CAD build for the part. Positions are in the model's coordinates, mm. Round coordinates to 2 decimals unless told otherwise and drop trailing zeros. Loops run counter-clockwise (first coordinate to the right, second up) from the corner with the lowest first, then second, coordinate; pieces in that order, holes last. Notation, with made-up numbers: (50, 7.25) - (59, 7.25) arc R30 ccw to (59, 42.25) - close; hole circle Ø6 at (68, 20.25). An arc over 180 degrees is marked (long way). One line per question, with ' | ' between items.
```python
from build123d import *

# Parameters (mm, degrees)
SKETCH_1_W            = 74
SKETCH_1_H            = 50
EXTRUDE_1_DEPTH       = 4
CUT_EXTRUDE_1_DEPTH   = 63.787339488
MIRROR_2_COPY_1_DEPTH = 63.787339488
SKETCH_3_R            = 13
CUT_EXTRUDE_2_DEPTH   = 63.787339488
FILLET_1_R            = 10
SKETCH_4_W            = 84
SKETCH_4_H            = 62
EXTRUDE_2_DEPTH       = 4
SKETCH_6_W            = 18
SKETCH_6_H            = 44
EXTRUDE_3_DEPTH       = 4
SKETCH_7_W            = 64
SKETCH_7_H            = 22
CUT_EXTRUDE_4_DEPTH   = 125.049385327
SKETCH_8_R            = 1.5
CUT_EXTRUDE_5_DEPTH   = 125.049385327
SKETCH_9_R            = 1.5
CUT_EXTRUDE_6_DEPTH   = 125.049385327
SKETCH_10_R           = 1.5
CUT_EXTRUDE_7_DEPTH   = 125.049385327
FILLET_2_R            = 3
SKETCH_11_W           = 20
SKETCH_11_H           = 18
CUT_EXTRUDE_8_DEPTH   = 125.049385327
FILLET_3_R            = 3
SKETCH_12_W           = 122.856865441
SKETCH_12_H           = 61.545901124
CUT_EXTRUDE_9_DEPTH   = 125.049385327
FILLET_4_R            = 3
FILLET_5_R            = 3
SKETCH_13_R           = 1.5
CUT_EXTRUDE_10_DEPTH  = 92.149602303
SKETCH_14_W           = 150.805924756
SKETCH_14_H           = 61.126695491
CUT_EXTRUDE_11_DEPTH  = 92.149602303
FILLET_6_R            = 1


with BuildPart() as part:
    # 草图1 → 凸台-拉伸1 (new body)
    with BuildSketch(Plane.XY):
        Polygon((37, 25), (42, 46.5), (-42, 46.5), (-37, 25), align=None)
        Rectangle(SKETCH_1_W, SKETCH_1_H)
    extrude(amount=EXTRUDE_1_DEPTH)

    # 草图2 → 切除-拉伸1 (cut, through all)
    with BuildSketch(Plane.XY.offset(4)):
        with BuildLine():
            ThreePointArc((29.5, 15), (29.939339828, 13.939339828), (31, 13.5))
            Line((31, 13.5), (31, 15))
            Line((31, 15), (29.5, 15))
        make_face()
        with BuildLine():
            Line((31, 15), (31, 13.5))
            ThreePointArc((31, 13.5), (32.060660172, 13.939339828), (32.5, 15))
            ThreePointArc((32.5, 15), (31, 16.5), (29.5, 15))
            Line((29.5, 15), (31, 15))
        make_face()
    cut_extrude_1 = extrude(amount=-CUT_EXTRUDE_1_DEPTH, mode=Mode.SUBTRACT)

    # 镜向1: 切除-拉伸1 across plane
    add(cut_extrude_1.mirror(Plane.ZX), mode=Mode.SUBTRACT)

    # 镜向2: 切除-拉伸1 across plane
    add(cut_extrude_1.mirror(Plane(origin=(0, 0, 0), x_dir=(0, 0, 1), z_dir=(1, 0, 0))), mode=Mode.SUBTRACT)

    # 镜向2 copy 1 sketch → 镜向2 copy 1 (cut, through all)
    with BuildSketch(Plane(origin=(0, 0, 4), x_dir=(-1, 0, 0), z_dir=(0, 0, 1))):
        with BuildLine():
            ThreePointArc((29.5, 15), (29.939339828, 13.939339828), (31, 13.5))
            Line((31, 13.5), (31, 15))
            Line((31, 15), (29.5, 15))
        make_face()
        with BuildLine():
            Line((31, 15), (31, 13.5))
            ThreePointArc((31, 13.5), (32.060660172, 13.939339828), (32.5, 15))
            ThreePointArc((32.5, 15), (31, 16.5), (29.5, 15))
            Line((29.5, 15), (31, 15))
        make_face()
    extrude(amount=-MIRROR_2_COPY_1_DEPTH, mode=Mode.SUBTRACT)

    # 草图3 → 切除-拉伸2 (cut, through all)
    with BuildSketch(Plane.XY.offset(4)):
        Circle(SKETCH_3_R)
    extrude(amount=-CUT_EXTRUDE_2_DEPTH, mode=Mode.SUBTRACT)

    # 圆角1
    fillet_1_edges = [part.edges().sort_by_distance(p)[0] for p in [
        (37, 25, 2),
        (-37, 25, 2),
    ]]
    fillet(fillet_1_edges, radius=FILLET_1_R)

    # 草图4 → 凸台-拉伸2 (add)
    with BuildSketch(Plane.XY.offset(4)):
        with Locations((0, 77.5)):
            Rectangle(SKETCH_4_W, SKETCH_4_H)
    extrude(amount=-EXTRUDE_2_DEPTH)

    # 草图6 → 凸台-拉伸3 (add)
    with BuildSketch(Plane.XY.offset(4)):
        with Locations((-51, 68.5)):
            Rectangle(SKETCH_6_W, SKETCH_6_H)
    extrude_3 = extrude(amount=-EXTRUDE_3_DEPTH)

    # 镜向4: 凸台-拉伸3 across plane
    add(extrude_3.mirror(Plane(origin=(0, 0, 0), x_dir=(0, 0, 1), z_dir=(1, 0, 0))))

    # 草图7 → 切除-拉伸4 (cut, through all)
    with BuildSketch(Plane.XY.offset(4)):
        with Locations((0, 69.5)):
            Rectangle(SKETCH_7_W, SKETCH_7_H)
    extrude(amount=-CUT_EXTRUDE_4_DEPTH, mode=Mode.SUBTRACT)

    # 草图8 → 切除-拉伸5 (cut, through all)
    with BuildSketch(Plane.XY.offset(4)):
        with Locations((0, 101)):
            Circle(SKETCH_8_R)
        with Locations((-24, 101)):
            Circle(SKETCH_8_R)
    cut_extrude_5 = extrude(amount=-CUT_EXTRUDE_5_DEPTH, mode=Mode.SUBTRACT)

    # 镜向5: 切除-拉伸5 across plane
    add(cut_extrude_5.mirror(Plane(origin=(0, 0, 0), x_dir=(0, 0, 1), z_dir=(1, 0, 0))), mode=Mode.SUBTRACT)

    # 草图9 → 切除-拉伸6 (cut, through all)
    with BuildSketch(Plane(origin=(0, 0, 0), x_dir=(-1, 0, 0), z_dir=(0, 0, -1))):
        with Locations((-52.5, 83.5)):
            Circle(SKETCH_9_R)
        with Locations((-52.5, 61)):
            Circle(SKETCH_9_R)
    cut_extrude_6 = extrude(amount=-CUT_EXTRUDE_6_DEPTH, mode=Mode.SUBTRACT)

    # 镜向6: 切除-拉伸6 across plane
    add(cut_extrude_6.mirror(Plane(origin=(0, 0, 0), x_dir=(0, 0, 1), z_dir=(1, 0, 0))), mode=Mode.SUBTRACT)

    # 草图10 → 切除-拉伸7 (cut, through all)
    with BuildSketch(Plane(origin=(0, 0, 0), x_dir=(-1, 0, 0), z_dir=(0, 0, -1))):
        with Locations((-30, 36)):
            Circle(SKETCH_10_R)
    cut_extrude_7 = extrude(amount=-CUT_EXTRUDE_7_DEPTH, mode=Mode.SUBTRACT)

    # 镜向7: 切除-拉伸7 across plane
    add(cut_extrude_7.mirror(Plane(origin=(0, 0, 0), x_dir=(0, 0, 1), z_dir=(1, 0, 0))), mode=Mode.SUBTRACT)

    # 圆角2
    fillet_2_edges = [part.edges().sort_by_distance(p)[0] for p in [
        (32, 80.5, 2),
        (32, 58.5, 2),
        (-32, 58.5, 2),
        (-32, 80.5, 2),
        (-42, 46.5, 2),
        (42, 46.5, 2),
        (-42, 90.5, 2),
        (42, 90.5, 2),
    ]]
    fillet(fillet_2_edges, radius=FILLET_2_R)

    # 草图11 → 切除-拉伸8 (cut, through all)
    with BuildSketch(Plane(origin=(0, 0, 0), x_dir=(-1, 0, 0), z_dir=(0, 0, -1))):
        with Locations((-50, 99.5)):
            Rectangle(SKETCH_11_W, SKETCH_11_H)
    cut_extrude_8 = extrude(amount=-CUT_EXTRUDE_8_DEPTH, mode=Mode.SUBTRACT)

    # 镜向8: 切除-拉伸8 across plane
    add(cut_extrude_8.mirror(Plane(origin=(0, 0, 0), x_dir=(0, 0, 1), z_dir=(1, 0, 0))), mode=Mode.SUBTRACT)

    # 圆角3
    fillet_3_edges = [part.edges().sort_by_distance(p)[0] for p in [
        (40, 90.5, 2),
        (-40, 90.5, 2),
    ]]
    fillet(fillet_3_edges, radius=FILLET_3_R)

    # 草图12 → 切除-拉伸9 (cut, through all)
    with BuildSketch(Plane(origin=(0, 0, 0), x_dir=(-1, 0, 0), z_dir=(0, 0, -1))):
        with Locations((1.42843272, 99.272950562)):
            Rectangle(SKETCH_12_W, SKETCH_12_H)
    extrude(amount=-CUT_EXTRUDE_9_DEPTH, mode=Mode.SUBTRACT)

    # 圆角4
    fillet_4_edges = [part.edges().sort_by_distance(p)[0] for p in [
        (-32, 68.5, 2),
        (32, 68.5, 2),
    ]]
    fillet(fillet_4_edges, radius=FILLET_4_R)

    # 圆角5
    fillet_5_edges = [part.edges().sort_by_distance(p)[0] for p in [
        (37, -25, 2),
        (-37, -25, 2),
    ]]
    fillet(fillet_5_edges, radius=FILLET_5_R)

    # 草图13 → 切除-拉伸10 (cut, through all)
    with BuildSketch(Plane.XY.offset(4)):
        with Locations((0, 36)):
            Circle(SKETCH_13_R)
    extrude(amount=-CUT_EXTRUDE_10_DEPTH, mode=Mode.SUBTRACT)

    # 草图14 → 切除-拉伸11 (cut, through all)
    with BuildSketch(Plane.XY.offset(4)):
        with Locations((-9.796052063, 74.063347746)):
            Rectangle(SKETCH_14_W, SKETCH_14_H)
    extrude(amount=-CUT_EXTRUDE_11_DEPTH, mode=Mode.SUBTRACT)

    # 圆角6
    fillet_6_edges = [part.edges().sort_by_distance(p)[0] for p in [
        (-41.302325581, 43.5, 2),
        (41.302325581, 43.5, 2),
    ]]
    fillet(fillet_6_edges, radius=FILLET_6_R)


solid = part.part
```
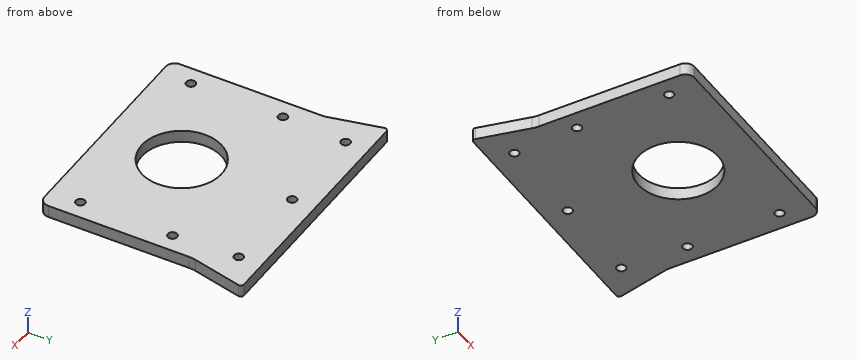
(1) Cut at B-B, the plane z = 1.05. State how many separate pieces and enclosed holes the cut face has, then the cut area to 3 significant figures.
Results found:
separate pieces: 1 | enclosed holes: 8 | area: 4,560 mm²
(2) Cut at A-A, the plane y = 0. Write the cut outline in (x, z).
Results found:
outline: (-37, 0) - (-13, 0) - (-13, 4) - (-37, 4) - close; (13, 0) - (37, 0) - (37, 4) - (13, 4) - close
(3) Probe L1, parallel to Y at x = 0, z = 0.65; L2, parallel to Y at x = -30, z = 2.45; L3, parallel to X at y = 8.5, z = 3.5. List the from-to ranges inside material, lowest first.
Results found:
L1: y = -25 to -13, 13 to 34.5, 37.5 to 43.5 | L2: y = -25 to -16.12, -13.88 to 13.88, 16.12 to 34.5, 37.5 to 43.5 | L3: x = -37 to -9.84, 9.84 to 37
(4) Drop a flat-ended pin along its axis: P1, Ø1, axis at y = 6.5, z = 3.5, coming from the -X side. Give the stop position or say it passes through.
Results found:
P1: stops at x = -37
(5) Cut at D-D, the plane y = 36. Write the cut outline in (x, z), then the cut area to 3 significant figures.
Results found:
outline: (-39.56, 0) - (-31.5, 0) - (-31.5, 4) - (-39.56, 4) - close; (-28.5, 0) - (-1.5, 0) - (-1.5, 4) - (-28.5, 4) - close; (1.5, 0) - (28.5, 0) - (28.5, 4) - (1.5, 4) - close; (31.5, 0) - (39.56, 0) - (39.56, 4) - (31.5, 4) - close | area: 280 mm²
(6) Cut at C-C, the plane x = 0. Write the cut outline in (y, z), then the cut area to 3 significant figures.
Results found:
outline: (-25, 0) - (-13, 0) - (-13, 4) - (-25, 4) - close; (13, 0) - (34.5, 0) - (34.5, 4) - (13, 4) - close; (37.5, 0) - (43.5, 0) - (43.5, 4) - (37.5, 4) - close | area: 158 mm²
